Verification items for the finished model (mm, model axes). Face numbers are marked on the shaded views. A direction names the side the tool comes from. Round coordinates to 2 decimals unless told otherwise and drop trailing zeros. Loops run counter-clockwise (first coordinate to the right, second up) from the corner with the lowest first, then second, coordinate; pieces in that order, holes last. Notation, with made-up numbers: M 5,39 L 57,39 A15 cw 57,45 Z; hole C 27,53.5 d11. An arc over 180 degrees is marked long. Answer as CSV lines item,"result".
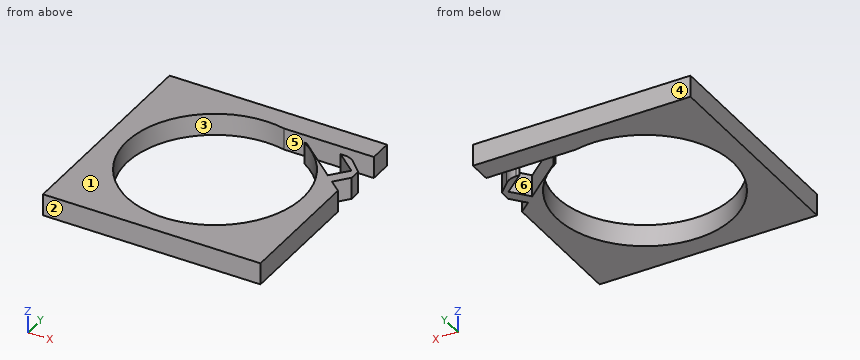
```python
from build123d import *

# Parameters (mm, degrees)
SKETCH1_W           = 127
SKETCH1_H           = 127
BOSS_EXTRUDE1_DEPTH = 12.7
CUT_EXTRUDE1_REACH  = 92.696
SKETCH2_R           = 51.5
CUT_EXTRUDE2_REACH  = 92.696
CUT_EXTRUDE3_REACH  = 92.696
CUT_EXTRUDE4_DEPTH  = 91.696141042
FILLET1_R           = 10


with BuildPart() as part:
    # Sketch1 → Boss-Extrude1 (new body)
    with BuildSketch(Plane.XY):
        Rectangle(SKETCH1_W, SKETCH1_H)
    extrude(amount=BOSS_EXTRUDE1_DEPTH)

    # Sketch2 → Cut-Extrude1 (cut, up to next)
    with BuildSketch(Plane.XY.offset(12.7), mode=Mode.PRIVATE) as cut_extrude1_sk1:
        Circle(SKETCH2_R)
    cut_extrude1_tool1 = extrude(cut_extrude1_sk1.sketch, amount=-CUT_EXTRUDE1_REACH, mode=Mode.PRIVATE) & part.part
    add(cut_extrude1_tool1.solids().sort_by_distance((0, 0, 12.7))[0], mode=Mode.SUBTRACT)

    # Sketch3 → Cut-Extrude2 (cut, up to next)
    with BuildSketch(Plane.XY.offset(12.7), mode=Mode.PRIVATE) as cut_extrude2_sk1:
        Polygon((0, 50.285247175), (63.5, 50.285247175), (63.5, 34.489292445), (48.70404527, 49.285247175), (0, 49.285247175), align=None)
    cut_extrude2_tool1 = extrude(cut_extrude2_sk1.sketch, amount=-CUT_EXTRUDE2_REACH, mode=Mode.PRIVATE) & part.part
    add(cut_extrude2_tool1.solids().sort_by_distance((31.75, 49.630895, 12.7))[0], mode=Mode.SUBTRACT)

    # Sketch4 → Cut-Extrude3 (cut, up to next)
    with BuildSketch(Plane.XY.offset(12.7), mode=Mode.PRIVATE) as cut_extrude3_sk1:
        Polygon((41.495660788, 49.285247175), (60.075181823, 33.695177927), (51.91177918, 23.9664135), (21.737968187, 49.285247175), align=None)
    cut_extrude3_tool1 = extrude(cut_extrude3_sk1.sketch, amount=-CUT_EXTRUDE3_REACH, mode=Mode.PRIVATE) & part.part
    # Sketch4 → Cut-Extrude3 (cut, up to next)
    with BuildSketch(Plane.XY.offset(12.7), mode=Mode.PRIVATE) as cut_extrude3_sk2:
        Polygon((56.676941472, 19.967967578), (63.5, 28.099372092), (63.5, 14.242741684), align=None)
    cut_extrude3_tool2 = extrude(cut_extrude3_sk2.sketch, amount=-CUT_EXTRUDE3_REACH, mode=Mode.PRIVATE) & part.part
    add(cut_extrude3_tool1.solids().sort_by_distance((43.251809, 38.865217, 12.7))[0], mode=Mode.SUBTRACT)
    add(cut_extrude3_tool2.solids().sort_by_distance((61.225647, 20.770027, 12.7))[0], mode=Mode.SUBTRACT)

    # Sketch5 → Cut-Extrude4 (cut, through all)
    with BuildSketch(Plane.XY.offset(12.7)):
        Polygon((11.794347458, 49.797355322), (57.138646711, 49.797355322), (57.138646711, 44.171093993), (19.361103765, 44.171093993), align=None)
    extrude(amount=-CUT_EXTRUDE4_DEPTH, mode=Mode.SUBTRACT)

    # Fillet1
    fillet1_edges = [part.edges().sort_by_distance(p)[0] for p in [
        (53.818198452, 44.171093993, 6.35),
    ]]
    fillet(fillet1_edges, radius=FILLET1_R)


solid = part.part
```
1) Material ranges on probe 1 along X at (y, z) = (0, 7.25); probe 2 along X at (y, z) = (26.5, 5.25), recorded low to high.
Here are the results:
probe 1,"x = -63.5 to -51.5, 51.5 to 63.5"
probe 2,"x = -63.5 to -44.16, 44.16 to 48.89, 54.04 to 62.16"
2) Section check C-C (z = 4). Record the cut outline in (x, y).
Here are the results:
outline,"M -63.5,-63.5 L 63.5,-63.5 L 63.5,14.24 L 56.68,19.97 L 63.5,28.1 L 63.5,34.49 L 56.75,41.24 A10 ccw 49.68,44.17 L 47.59,44.17 L 60.08,33.7 L 51.91,23.97 L 27.83,44.17 L 26.48,44.17 A51.5 cw long 11.12,50.29 L 63.5,50.29 L 63.5,63.5 L -63.5,63.5 Z"
3) Section check D-D (x = 29.5). Record the cut outline in (y, z), plus the area to 3 significant figures.
Here are the results:
outline,"M -63.5,0 L -42.21,0 L -42.21,12.7 L -63.5,12.7 Z; M 42.21,0 L 42.77,0 L 42.77,12.7 L 42.21,12.7 Z; M 50.29,0 L 63.5,0 L 63.5,12.7 L 50.29,12.7 Z"
area,"445 mm^2"
4) Set-up check for the marked faces 4, 5 and 6: record each of +Z, -Z, +X, -X, +Y, -Y from which the full face is reachable in a straight line by a thin tool's end or side.
Here are the results:
face 4,"+Z, -Z, +X, -X, +Y"
face 5,"+Z, -Z, +X"
face 6,"+Z, -Z"
5) Section check A-A (x = 0). Record the cut outline in (y, z), plus the area to 3 significant figures.
Here are the results:
outline,"M -63.5,0 L -51.5,0 L -51.5,12.7 L -63.5,12.7 Z; M 51.5,0 L 63.5,0 L 63.5,12.7 L 51.5,12.7 Z"
area,"305 mm^2"
6) Draft check along Y on the marked faces 1, 2 and 3. Enter one of: +Y half, -Y half, draft (parallel to the pull), parting line (faces both ways), or undercut.
Here are the results:
face 1,"draft"
face 2,"-Y half"
face 3,"undercut"
